Build history of the part. All positions in model axes, mm. Face numbers are marked on the shaded views. Coordinates: 2 decimals unless noted, no trailing zeros. Loops run counter-clockwise (first coordinate to the right, second up) from the corner with the lowest first, then second, coordinate; pieces in that order, holes last.
(1) Slice it at B-B (y = 1.5). Give the number of separate pieces and of enclosed holes in the cut face, and give its area (3 significant figures).
(2) Wall check: L1, parallel to Z at x = 0, y = 0.8; L2, parallel to Y at x = 11.5, z = -2.25; L3, parallel to X at y = -0.85, z = -0.5. Give the ranges that are in metal, low to high.
(3) Flat gauge pins, fed straight in: P1, Ø1.3, axis at x = 0, z = -1, coming from the +Y side; P2, Ø2, axis at x = 12, z = -1, coming from the -Y side; P3, Ø2, axis at y = -0.5, z = 2.5, coming from the -X side. Where does each tip first touch, or does it go through?
(4) Slice it at A-A (x = 0). Give the cut face in (y, z).
(5) Two-plate mould, pull along Z, no slides. Class the marked faces 1, 2 and 3: pulls with the +Z half, pulls with the -Z half, needs draft (parallel to the pull), parting line crosses it, or undercut.
(6) Slice it at C-C (y = -0.45). Give the cut face in (x, z).
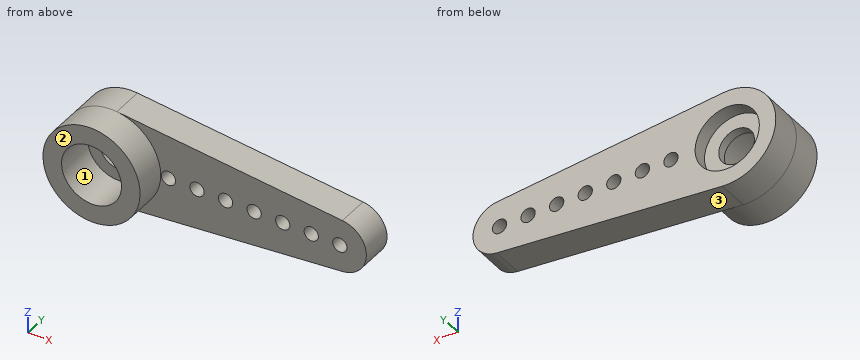
from build123d import *

# Parameters (mm, degrees)
BOSS_EXTRU_1_DEPTH              = 2.2
BOSS_EXTRU_2_START              = 2.2
ESQUISSE2_R                     = 3.4
BOSS_EXTRU_2_DEPTH              = 2.2
ESQUISSE3_R                     = 2.1
ENL_V_MAT_EXTRU_1_DEPTH         = 2.8
DIAM_TRE_DU_PER_AGE_2_5_2_5_1_D = 2.5
DIAM_TRE_DU_PER_AGE_1_0_1_1_D   = 1
ESQUISSE8_R                     = 2.25
ENL_V_MAT_EXTRU_2_DEPTH         = 1


with BuildPart() as part:
    # Esquisse1 → Boss.-Extru.1 (new body)
    with BuildSketch(Plane(origin=(0, 0, 0), x_dir=(1, 0, 0), z_dir=(0, 1, 0))):
        with BuildLine():
            Line((0.32873073, 3.384070937), (16.121002055, 1.85))
            ThreePointArc((16.121002055, 1.85), (17.8, 0), (16.121002055, -1.85))
            Line((16.121002055, -1.85), (0.32873073, -3.384070937))
            ThreePointArc((0.32873073, -3.384070937), (-3.4, 0), (0.32873073, 3.384070937))
        make_face()
    extrude(amount=BOSS_EXTRU_1_DEPTH)

    # Esquisse2 → Boss.-Extru.2 (add)
    with BuildSketch(Plane.XZ.offset(BOSS_EXTRU_2_START)):
        with Locations(Location((0, 0, 0), (0, 0, 270))):
            Circle(ESQUISSE2_R)
    extrude(amount=-BOSS_EXTRU_2_DEPTH)

    # Esquisse3 → Enlèv. mat.-Extru.1 (cut)
    with BuildSketch(Plane.XZ.offset(2.2)):
        with Locations(Location((0, 0, 0), (0, 0, 270))):
            Circle(ESQUISSE3_R)
    extrude(amount=-ENL_V_MAT_EXTRU_1_DEPTH, mode=Mode.SUBTRACT)

    # Diamètre du perçage Ø2.5 (2.5)1 (through all)
    with Locations(Plane(origin=(0, 2.2, 0), x_dir=(1, 0, 0), z_dir=(0, 1, 0))):
        with Locations((0, 0)):
            Hole(DIAM_TRE_DU_PER_AGE_2_5_2_5_1_D / 2)

    # Diamètre du perçage Ø1.0 (1)1 (through all)
    with Locations(Plane(origin=(0, 0, 0), x_dir=(-1, 0, 0), z_dir=(0, -1, 0))):
        with Locations((-15.941291918, 0), (-13.941291918, 0), (-11.941291918, 0), (-9.941291918, 0), (-7.941291918, 0), (-5.941291918, 0), (-3.941291918, 0)):
            Hole(DIAM_TRE_DU_PER_AGE_1_0_1_1_D / 2)

    # Esquisse8 → Enlèv. mat.-Extru.2 (cut)
    with BuildSketch(Plane(origin=(0, 2.2, 0), x_dir=(1, 0, 0), z_dir=(0, 1, 0))):
        with Locations(Location((0, 0, 0), (0, 0, 270))):
            Circle(ESQUISSE8_R)
    extrude(amount=-ENL_V_MAT_EXTRU_2_DEPTH, mode=Mode.SUBTRACT)


solid = part.part
Response values:
1. separate pieces: 1
1. enclosed holes: 8
1. area: 86.4 mm2
2. L1: z = -3.4 to -1.25, 1.25 to 3.4
2. L2: y = 0 to 2.2
2. L3: x = -3.36 to -2.04, 2.04 to 3.36
3. P1: stops at y = 1.2
3. P2: stops at y = 0
3. P3: stops at x = -3.05
4. outline: (-2.2, -3.4) - (2.2, -3.4) - (2.2, -2.25) - (1.2, -2.25) - (1.2, -1.25) - (0.6, -1.25) - (0.6, -2.1) - (-2.2, -2.1) - close; (-2.2, 2.1) - (0.6, 2.1) - (0.6, 1.25) - (1.2, 1.25) - (1.2, 2.25) - (2.2, 2.25) - (2.2, 3.4) - (-2.2, 3.4) - close
5. face 1: undercut
5. face 2: needs draft
5. face 3: pulls with the -Z half
6. outline: circle Ø6.8 at (0, 0); hole circle Ø4.2 at (0, 0)
